```python
from build123d import *

# Parameters (mm, degrees)
ESBO_O1_R                = 5.5
ESBO_O1_R_2              = 2
RESSALTO_EXTRUS_O1_DEPTH = 9.7
ESBO_O2_R                = 8.5
ESBO_O2_R_2              = 2.8
RESSALTO_EXTRUS_O2_DEPTH = 5.3


with BuildPart() as part:
    # Esboço1 → Ressalto-extrusão1 (new body)
    with BuildSketch(Plane.XY):
        with BuildLine():
            Line((-12.397968723, -0.166390596), (-11.838135129, -41.880282782))
            ThreePointArc((-11.838135129, -41.880282782), (-5.631724082, -48.255001448), (1.066308546, -42.398984451))
            Line((1.066308546, -42.398984451), (3.948309434, -11.753644835))
            ThreePointArc((3.948309434, -11.753644835), (7.17044634, 10.115434423), (-12.397968723, -0.166390596))
        make_face()
        Circle(ESBO_O1_R, mode=Mode.SUBTRACT)
        with Locations((-5.372000333, -41.793502112)):
            Circle(ESBO_O1_R_2, mode=Mode.SUBTRACT)
    extrude(amount=RESSALTO_EXTRUS_O1_DEPTH)

    # Esboço2 → Ressalto-extrusão2 (add)
    with BuildSketch(Plane.XY.offset(9.7)):
        Circle(ESBO_O2_R)
        Circle(ESBO_O2_R_2, mode=Mode.SUBTRACT)
    extrude(amount=RESSALTO_EXTRUS_O2_DEPTH)


solid = part.part
```
Input: part model. Units: mm. Frame: model coordinates. A direction names the side the tool comes from. Coordinates: 2 decimals unless noted, no trailing zeros. Write each loop counter-clockwise with the first axis right and the second up, starting at its lowest first coordinate (ties: lowest second). Pieces come first, ordered by that corner, then holes.
1) Section D-D on z = 7. Output: boundary loops of the cut face in (x, y), and give its area (3 significant figures).
2) Section C-C on x = 4.5. Output: boundary loops of the cut face in (y, z), and give its area (3 significant figures).
3) Set-up query: faces 1 (the flat face through (-3, 1, 9.7)), 2 (the cylindrical face through (4.57, 7.167, 12.313)), 3 (the flat face through (4, 0, 15)). Return all of +Z, -Z, +X, -X, +Y, -Y with unobstructed straight access to the full face (end or side cutting, diameter ignored); none if empty.
4) Section B-B on x = 0. Output: boundary loops of the cut face in (y, z).
5) Pin query (flat end, axial travel): pin 1 Ø10 at (x, y) = (-3, -28) entering from +Z; pin 2 Ø1 at (y, z) = (-11, 2) entering from -X; pin 3 Ø1 at (x, z) = (0.5, 6) entering from -Y; pin 4 Ø12 at (x, y) = (-2, 0) entering from -Z. Return the tip coordinate at first contact, or that it passes through.
6) Section A-A on z = 12. Output: boundary loops of the cut face in (x, y).
7) Material intervals for line 1 along Y through (x, z) = (0, 11.6); line 2 along Z through (x, y) = (-1.5, -23); line 3 along Y through (x, z) = (0, 7.25), sorted ascending.
Check result:
1. outline: (-12.4, -0.17) - (-11.84, -41.88) arc R6.47 ccw to (1.07, -42.4) - (3.95, -11.75) arc R12.4 ccw (long way) to start; hole circle Ø4 at (-5.37, -41.79); hole circle Ø11 at (0, 0)
1. area: 901 mm2
2. outline: (-11.55, 0) - (-3.16, 0) - (-3.16, 9.7) - (3.16, 9.7) - (3.16, 0) - (11.55, 0) - (11.55, 9.7) - (7.21, 9.7) - (7.21, 15) - (-7.21, 15) - (-7.21, 9.7) - (-11.55, 9.7) - close
2. area: 239 mm2
3. face 1: -Z
3. face 2: +Z
3. face 3: +Z, +X, -X, +Y, -Y
4. outline: (-45.39, 0) - (-5.5, 0) - (-5.5, 9.7) - (-2.8, 9.7) - (-2.8, 15) - (-8.5, 15) - (-8.5, 9.7) - (-45.39, 9.7) - close; (2.8, 9.7) - (5.5, 9.7) - (5.5, 0) - (12.4, 0) - (12.4, 9.7) - (8.5, 9.7) - (8.5, 15) - (2.8, 15) - close
5. pin 1: stops at z = 9.7
5. pin 2: stops at x = -12.26
5. pin 3: stops at y = -45.39
5. pin 4: stops at z = 0
6. outline: circle Ø17 at (0, 0); hole circle Ø5.6 at (0, 0)
7. line 1: y = -8.5 to -2.8, 2.8 to 8.5
7. line 2: z = 0 to 9.7
7. line 3: y = -45.39 to -5.5, 5.5 to 12.4
